Source: CAD feature listing. Evaluate the final solid. Frame: model axes, mm. Face numbers are marked on the shaded views. Round coordinates to 2 decimals unless told otherwise and drop trailing zeros. Order: outer loops, then holes, each group sorted by start corner. A loop starts at its lowest first (then second) coordinate and runs counter-clockwise, first axis right, second up. Notation, with made-up numbers: M 45.5,54.5 L 50.5,54.5 A27 cw 50.5,75.5 Z; hole C 2.5,36.5 d10. An arc over 180 degrees is marked long. Answer in a Markdown table with one row per item. Add a question column.
```python
from build123d import *

# Parameters (mm, degrees)
PAD_DEPTH    = 10
SKETCH001_W  = 101.6
SKETCH001_H  = 53.3
POCKET_DEPTH = 7
SKETCH002_R  = 2
PAD001_DEPTH = 2


with BuildPart() as part:
    # Sketch → Pad (new body)
    with BuildSketch(Plane.XY):
        with BuildLine():
            ThreePointArc((0, 55.3), (-1.414219, 54.714208), (-2, 53.299986))
            Line((-2, 0), (-2, 53.299986))
            ThreePointArc((-2, 0), (-1.414214, -1.414214), (0, -2))
            Line((101.6, -2), (0, -2))
            ThreePointArc((101.6, -2), (103.014214, -1.414214), (103.6, 0))
            Line((103.6, 53.3), (103.6, 0))
            ThreePointArc((103.6, 53.3), (103.014214, 54.714214), (101.6, 55.3))
            Line((0, 55.3), (101.6, 55.3))
        make_face()
    extrude(amount=PAD_DEPTH)

    # Sketch001 → Pocket (cut)
    with BuildSketch(Plane.XY.offset(10)):
        with Locations((50.786842, 26.274506)):
            Rectangle(SKETCH001_W, SKETCH001_H)
    extrude(amount=-POCKET_DEPTH, mode=Mode.SUBTRACT)

    # Sketch002 → Pad001 (new body)
    with BuildSketch(Plane.XY.offset(3)):
        with Locations((15.3, 50.7)):
            Circle(SKETCH002_R)
        with Locations((14, 2.5)):
            Circle(SKETCH002_R)
        with Locations((66.1, 35.5)):
            Circle(SKETCH002_R)
        with Locations((66.1, 7.6)):
            Circle(SKETCH002_R)
        with Locations((90.2, 50.7)):
            Circle(SKETCH002_R)
        with Locations((95.2, 2.5)):
            Circle(SKETCH002_R)
    extrude(amount=PAD001_DEPTH)


solid = part.part
```
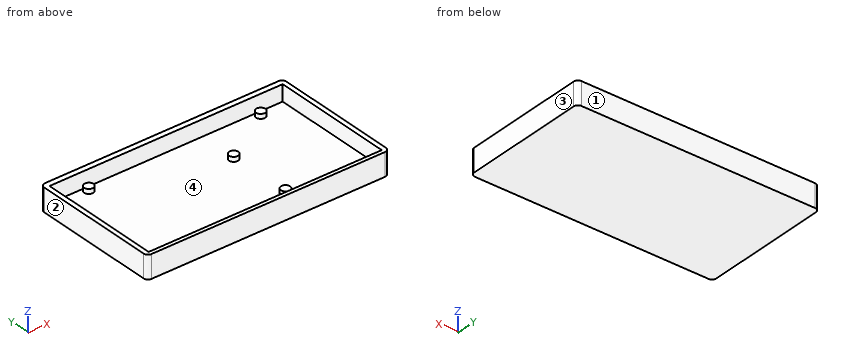
(1) Draft query along X for the marked faces 1, 2, 3 and 4. Return one class per face: +X half, -X half, draft (parallel to the pull), parting line (faces both ways), or undercut.
(2) Pin query (flat end, axial travel): pin 1 (1 mm diameter, centred on x = 43, y = 19.5, fed in from +Z); pin 2 (3 mm diameter, centred on x = 14, y = 2.5, fed in from +Z). Return the tip coordinate at first contact, or that it passes through.
(3) Cut plane D-D (y = 43). Return loops of the section in (x, z), and give its area (3 significant figures).
(4) Line query: line 1 (Y direction, x = 95.5, z = 4.5); line 2 (X direction, y = 45.5, z = 8); line 3 (Y direction, x = 43, z = 8). Output: solid intervals per line, ascending. Write a range as from..to.
(5) Cut plane A-A (z = 8). Return loops of the section in (x, y).
(6) Cut plane B-B (x = 90.2). Return loops of the section in (y, z), and give its area (3 significant figures).
(7) Cut plane C-C (y = 7.6). Return loops of the section in (x, z).
Answer list:
| question | item | result |
|---|---|---|
| 1 | face 1 | draft |
| 1 | face 2 | -X half |
| 1 | face 3 | +X half |
| 1 | face 4 | undercut |
| 2 | pin 1 | z = 3 |
| 2 | pin 2 | z = 5 |
| 3 | outline | M -2,0 L 103.6,0 L 103.6,10 L 101.59,10 L 101.59,3 L -0.01,3 L -0.01,10 L -2,10 Z |
| 3 | area | 345 mm² |
| 4 | line 1 | -2..-0.38, 0.52..4.48, 52.92..55.3 |
| 4 | line 2 | -2..-0.01, 101.59..103.6 |
| 4 | line 3 | -2..-0.38, 52.92..55.3 |
| 5 | outline | M -2,0 A2 ccw 0,-2 L 101.6,-2 A2 ccw 103.6,0 L 103.6,53.3 A2 ccw 101.6,55.3 L 0,55.3 A2 ccw -2,53.3 Z; hole M -0.01,-0.38 L 101.59,-0.38 L 101.59,52.92 L -0.01,52.92 Z |
| 6 | outline | M -2,0 L 55.3,0 L 55.3,10 L 52.92,10 L 52.92,3 L 52.7,3 L 52.7,5 L 48.7,5 L 48.7,3 L -0.38,3 L -0.38,10 L -2,10 Z |
| 6 | area | 208 mm² |
| 7 | outline | M -2,0 L 103.6,0 L 103.6,10 L 101.59,10 L 101.59,3 L 68.1,3 L 68.1,5 L 64.1,5 L 64.1,3 L -0.01,3 L -0.01,10 L -2,10 Z |
